For this review, take the finished solid that the model builds, in its own axes (mm). Give positions to 0.01 mm unless a question says otherwise; leave off trailing zeros. Loops run counter-clockwise (first coordinate to the right, second up) from the corner with the lowest first, then second, coordinate; pieces in that order, holes last. Notation, with made-up numbers: (45, 76.5) - (98, 76.5) arc R21 ccw to (98, 112.5) - close; hole circle Ø1 at (57.25, 66.5). An arc over 180 degrees is marked (long way). Put each result on its own line as item: value. Start each with the question number.
from build123d import *

# Parameters (mm, degrees)
BOSS_EXTRUDE1_DEPTH = 1.524


with BuildPart() as part:
    # Sketch1 → Boss-Extrude1 (new body)
    with BuildSketch(Plane.XY):
        with BuildLine():
            Line((150.036715568, -1.524), (150.036715568, 0))
            Line((150.036715568, 0), (119.605645903, 0))
            Line((119.605645903, 0), (143.313878366, 6.056634362))
            Line((143.313878366, 6.056634362), (142.879507781, 7.877232472))
            Line((142.879507781, 7.877232472), (149.056142524, 9.350895679))
            Line((149.056142524, 9.350895679), (149.467068546, 7.628561883))
            Line((149.467068546, 7.628561883), (187.215425718, 17.271963073))
            ThreePointArc((187.215425718, 17.271963073), (186.146982613, 8.178774912), (190.262232611, 0))
            Line((190.262232611, 0), (190.262232611, -1.524))
            ThreePointArc((190.262232611, -1.524), (186.146982613, -9.702774912), (187.215425718, -18.795963073))
            Line((187.215425718, -18.795963073), (149.467068546, -9.152561883))
            Line((149.467068546, -9.152561883), (149.056142524, -10.874895679))
            Line((149.056142524, -10.874895679), (142.879507781, -9.401232472))
            Line((142.879507781, -9.401232472), (143.313878366, -7.580634362))
            Line((143.313878366, -7.580634362), (119.605645903, -1.524))
            Line((119.605645903, -1.524), (150.036715568, -1.524))
        make_face()
    extrude(amount=BOSS_EXTRUDE1_DEPTH)


solid = part.part
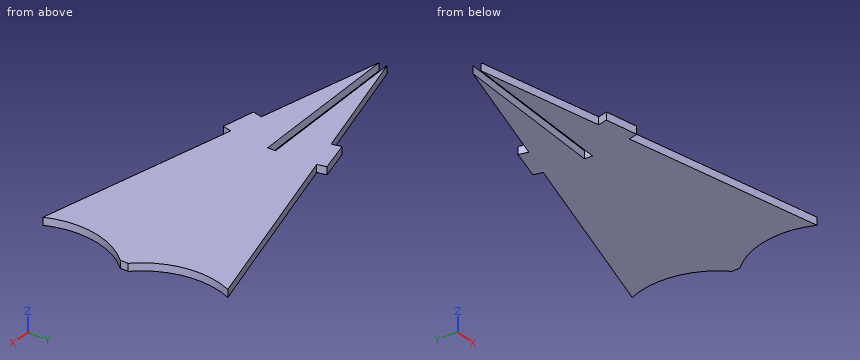
1) Take a section at C-C on x = 147.5. State the section outline as (y, z) points.
2) Take a section at D-D on y = -8.5. State the section outline as (x, z) points.
3) Take a section at B-B on z = 1.1. State the section outline as (x, y) points, and give its area (3 significant figures).
4) Wall thickness on probe 1 along X at (y, z) = (-1, 0.95); probe 2 along Y at (x, z) = (130.5, 0.7); probe 3 along Y at (x, z) = (140.5, 0.4): over which ranges is each line inside the solid? List them lowest first.
5) Insertion check: P1, Ø0.5, axis at x = 135.5, z = 0.5, coming from the -Y side; P2, Ø0.5, axis at y = -1, z = 0.5, coming from the -X side. Each pin has a flat end and moves straight along its axis. Give the tip position at first contact, or say it passes through.
6) Take a section at A-A on x = 137. State the section outline as (y, z) points.
Answers follow:
1. outline: (-10.5, 0) - (-1.52, 0) - (-1.52, 1.52) - (-10.5, 1.52) - close; (0, 0) - (8.98, 0) - (8.98, 1.52) - (0, 1.52) - close
2. outline: (143.09, 0) - (186.41, 0) - (186.41, 1.52) - (143.09, 1.52) - close
3. outline: (119.61, -1.52) - (143.31, -7.58) - (142.88, -9.4) - (149.06, -10.87) - (149.47, -9.15) - (187.22, -18.8) arc R15.93 cw to (190.26, -1.52) - (190.26, 0) arc R15.93 cw to (187.22, 17.27) - (149.47, 7.63) - (149.06, 9.35) - (142.88, 7.88) - (143.31, 6.06) - (119.61, 0) - (150.04, 0) - (150.04, -1.52) - close
3. area: 1,240 mm2
4. probe 1: 150.04 to 190.26
4. probe 2: -4.31 to -1.52, 0 to 2.78
4. probe 3: -6.86 to -1.52, 0 to 5.34
5. P1: y = -5.65
5. P2: x = 150.04
6. outline: (-5.97, 0) - (-1.52, 0) - (-1.52, 1.52) - (-5.97, 1.52) - close; (0, 0) - (4.44, 0) - (4.44, 1.52) - (0, 1.52) - close
